Verification items for the finished model (mm, model axes). A direction names the side the tool comes from. Coordinates: 2 decimals unless noted, no trailing zeros. Order: outer loops, then holes, each group sorted by start corner. A loop starts at its lowest first (then second) coordinate and runs counter-clockwise, first axis right, second up.
Q1. Thickness scan on line 1 (X direction, y = -85, z = 5.25); line 2 (Z direction, x = -12, y = -46); line 3 (X direction, y = -49, z = 4.25). Record the ranges inside material, lowest first.
Q2. Draft check along Z on faces 1 (the flat face through (0, 48, -7.5)), 2 (the flat face through (0, -46, -0.5)), 3 (the flat face through (0, -44.031, -5)). Enter one of: pulls with the +Z half, pulls with the -Z half, needs draft (parallel to the pull), parting line crosses it, or undercut.
Q3. Depth check by flat-ended pin: P1, Ø3.5, axis at x = -7.5, y = -44, coming from the +Z side; P2, Ø2, axis at y = -70.5, z = 7, coming from the -X side; P3, Ø1, axis at x = -25.5, z = 1, coming from the -Y side. Enter the tip coordinate at first touch or a pass-through.
Q4. Cross-section at A-A, the plane y = 9.5. Record the boundary of the cut face in (x, z).
Q5. Set-up check for faces 4 (the flat face through (-17.363, 42, 0)), 5 (the cylindrical face through (-25.937, 24.446, -0.133)), 6 (the cylindrical face through (-10, 48, 0)), 7 (the flat face through (-20, -86, 0)): record each of +Z, -Z, +X, -X, +Y, -Y from which the full face is reachable in a straight line by a thin tool's end or side.
Q6. Cross-section at B-B, the plane x = 24.5. Record the boundary of the cut face in (y, z), and give its area (3 significant figures).
from build123d import *

# Parameters (mm, degrees)
BOSS_EXTRUDE1_DEPTH  = 6.9
BOSS_EXTRUDE2_START  = -6.9
BOSS_EXTRUDE2_DEPTH  = 51.9
CUT_EXTRUDE1_DEPTH   = 50.160278182
BOSS_EXTRUDE4_START  = -6.9
BOSS_EXTRUDE4_DEPTH  = 6.9
BOSS_EXTRUDE5_DEPTH  = 19
BOSS_EXTRUDE8_DEPTH  = 19
CUT_EXTRUDE2_DEPTH   = 38.1
SKETCH16_W           = 3.4
SKETCH16_H           = 19
BOSS_EXTRUDE10_DEPTH = 68.4
BOSS_EXTRUDE11_DEPTH = 68.4
SKETCH18_W           = 40
SKETCH18_H           = 19
BOSS_EXTRUDE12_DEPTH = 5
CUT_EXTRUDE3_START   = -7.338241
SKETCH20_W           = 33.2
SKETCH20_H           = 10
CUT_EXTRUDE3_DEPTH   = 7.338241
BOSS_EXTRUDE13_DEPTH = 19
FILLET1_R            = 5
SKETCH22_R           = 2
CUT_EXTRUDE4_DEPTH   = 49.030762114


with BuildPart() as part:
    # Sketch1 → Boss-Extrude1 (new body)
    with BuildSketch(Plane(origin=(0, 0, 0), x_dir=(1, 0, 0), z_dir=(0, 1, 0))):
        with BuildLine():
            ThreePointArc((7.36326441, 9.5), (12.000269064, 0), (7.36326441, -9.5))
            Line((7.36326441, -9.5), (0, -9.5))
            Line((0, -9.5), (-7.36326441, -9.5))
            ThreePointArc((-7.36326441, -9.5), (-12.000269064, 0), (-7.36326441, 9.5))
            Line((-7.36326441, 9.5), (0, 9.5))
            Line((0, 9.5), (7.36326441, 9.5))
        make_face()
        with BuildLine():
            Line((0, 7.5), (6.64, 7.5))
            ThreePointArc((6.64, 7.5), (10.000269064, 0), (6.64, -7.5))
            Line((6.64, -7.5), (0, -7.5))
            Line((0, -7.5), (-6.64, -7.5))
            ThreePointArc((-6.64, -7.5), (-10.000269064, 0), (-6.64, 7.5))
            Line((-6.64, 7.5), (0, 7.5))
        make_face(mode=Mode.SUBTRACT)
    extrude(amount=BOSS_EXTRUDE1_DEPTH)

    # Sketch2 → Boss-Extrude2 (add)
    with BuildSketch(Plane(origin=(0, 6.9, 0), x_dir=(1, 0, 0), z_dir=(0, 1, 0)).offset(BOSS_EXTRUDE2_START)):
        with BuildLine():
            Line((-7.36326441, 9.5), (-17.36326441, 9.5))
            Line((-17.36326441, 9.5), (-17.36326441, -9.5))
            Line((-17.36326441, -9.5), (-7.36326441, -9.5))
            ThreePointArc((-7.36326441, -9.5), (-12.000269064, 0), (-7.36326441, 9.5))
        make_face()
    boss_extrude2 = extrude(amount=BOSS_EXTRUDE2_DEPTH)

    # Sketch4 → Cut-Extrude1 (cut, through all)
    with BuildSketch(Plane(origin=(0, 6.9, 0), x_dir=(1, 0, 0), z_dir=(0, 1, 0))):
        with BuildLine():
            Line((-10.915369405, -4.996906494), (-8.86326441, -9.5))
            Line((-8.86326441, -9.5), (-7.36326441, -9.5))
            ThreePointArc((-7.36326441, -9.5), (-9.411139164, -7.462870557), (-10.915369405, -4.996906494))
        make_face()
        with BuildLine():
            Line((-10.915369405, 4.996906494), (-8.86326441, 9.5))
            Line((-8.86326441, 9.5), (-7.36326441, 9.5))
            ThreePointArc((-7.36326441, 9.5), (-9.411139164, 7.462870557), (-10.915369405, 4.996906494))
        make_face()
    cut_extrude1 = extrude(amount=CUT_EXTRUDE1_DEPTH, mode=Mode.SUBTRACT)

    # Mirror2: Boss-Extrude2, Cut-Extrude1 across plane
    add(boss_extrude2.mirror(Plane(origin=(0, 0, 0), x_dir=(0, 0, 1), z_dir=(1, 0, 0))))
    add(cut_extrude1.mirror(Plane(origin=(0, 0, 0), x_dir=(0, 0, 1), z_dir=(1, 0, 0))), mode=Mode.SUBTRACT)

    # Sketch6 → Boss-Extrude4 (add)
    with BuildSketch(Plane(origin=(0, 51.9, 0), x_dir=(1, 0, 0), z_dir=(0, 1, 0)).offset(BOSS_EXTRUDE4_START)):
        with BuildLine():
            Line((10.915369405, 4.996906494), (8.86326441, 9.5))
            Line((8.86326441, 9.5), (-8.86326441, 9.5))
            Line((-8.86326441, 9.5), (-10.915369405, 4.996906494))
            ThreePointArc((-10.915369405, 4.996906494), (-12.000269064, 0), (-10.915369405, -4.996906494))
            Line((-10.915369405, -4.996906494), (-8.86326441, -9.5))
            Line((-8.86326441, -9.5), (8.86326441, -9.5))
            Line((8.86326441, -9.5), (10.915369405, -4.996906494))
            ThreePointArc((10.915369405, -4.996906494), (12.000269064, 0), (10.915369405, 4.996906494))
        make_face()
        with BuildLine():
            Line((-6.64, 7.5), (6.64, 7.5))
            ThreePointArc((6.64, 7.5), (10.000269064, 0), (6.64, -7.5))
            Line((6.64, -7.5), (-6.64, -7.5))
            ThreePointArc((-6.64, -7.5), (-10.000269064, 0), (-6.64, 7.5))
        make_face(mode=Mode.SUBTRACT)
    extrude(amount=BOSS_EXTRUDE4_DEPTH)

    # Sketch7 → Boss-Extrude5 (add)
    with BuildSketch(Plane.XY.offset(9.5)):
        Polygon((-17.36326441, 31.95), (-35, 31.95), (-35, -23.05), (-27.36326441, -23.05), (-27.36326441, 25.95), (-17.36326441, 25.95), align=None)
    boss_extrude5 = extrude(amount=-BOSS_EXTRUDE5_DEPTH)

    # Mirror4: Boss-Extrude5 across plane
    add(boss_extrude5.mirror(Plane(origin=(0, 0, 0), x_dir=(0, 0, 1), z_dir=(1, 0, 0))))

    # Sketch11 → Boss-Extrude8 (add)
    with BuildSketch(Plane.XY.offset(9.5)):
        Polygon((-35, -23.05), (-20, -49.030762114), (20, -49.030762114), (35, -23.05), (27.36326441, -23.05), (15.250015756, -44.030762114), (-15.250015756, -44.030762114), (-27.36326441, -23.05), align=None)
    extrude(amount=-BOSS_EXTRUDE8_DEPTH)

    # Sketch15 → Cut-Extrude2 (cut)
    with BuildSketch(Plane(origin=(0, 6.9, 0), x_dir=(1, 0, 0), z_dir=(0, 1, 0))):
        Polygon((-12.000269064, 0), (-12.000269064, 9.5), (12.000269064, 9.5), (12.000269064, 0), (12.000269064, -9.5), (-12.000269064, -9.5), align=None)
    extrude(amount=CUT_EXTRUDE2_DEPTH, mode=Mode.SUBTRACT)

    # Sketch16 → Boss-Extrude10 (add)
    with BuildSketch(Plane.XZ.offset(49.030762114)):
        with Locations((-18.3, 0)):
            Rectangle(SKETCH16_W, SKETCH16_H)
        with Locations((18.3, 0)):
            Rectangle(SKETCH16_W, SKETCH16_H)
    extrude(amount=BOSS_EXTRUDE10_DEPTH)

    # Sketch17 → Boss-Extrude11 (add)
    with BuildSketch(Plane.XZ.offset(49.030762114)):
        with BuildLine():
            Line((-14.6, -9.5), (-16.6, -9.5))
            Line((-16.6, -9.5), (-16.6, -7.5))
            ThreePointArc((-16.6, -7.5), (-16.014213562, -8.914213562), (-14.6, -9.5))
        make_face()
        with BuildLine():
            Line((14.6, -9.5), (16.6, -9.5))
            Line((16.6, -9.5), (16.6, -7.5))
            ThreePointArc((16.6, -7.5), (16.014213562, -8.914213562), (14.6, -9.5))
        make_face()
    extrude(amount=BOSS_EXTRUDE11_DEPTH)

    # Sketch18 → Boss-Extrude12 (add)
    with BuildSketch(Plane.XZ.offset(117.430762114)):
        Rectangle(SKETCH18_W, SKETCH18_H)
    extrude(amount=BOSS_EXTRUDE12_DEPTH)

    # Sketch20 → Cut-Extrude3 (cut)
    with BuildSketch(Plane.XZ.offset(49.030762114).offset(CUT_EXTRUDE3_START)):
        with Locations((0, 4.5)):
            Rectangle(SKETCH20_W, SKETCH20_H)
    extrude(amount=CUT_EXTRUDE3_DEPTH, mode=Mode.SUBTRACT)

    # Sketch21 → Boss-Extrude13 (add)
    with BuildSketch(Plane.XY.offset(9.5)):
        Polygon((-20, -122.430762114), (0, -197.071778265), (20, -122.430762114), align=None)
    extrude(amount=-BOSS_EXTRUDE13_DEPTH)

    # Fillet1
    fillet1_edges = [part.edges().sort_by_distance(p)[0] for p in [
        (20, -122.430762114, 0),
        (20, -49.030762114, 0),
        (35, -23.05, 0),
        (35, 31.95, 0),
        (17.36326441, 31.95, 0),
        (-17.36326441, 31.95, 0),
        (-35, 31.95, 0),
        (-35, -23.05, 0),
        (-20, -49.030762114, 0),
        (-20, -122.430762114, 0),
        (-17.36326441, 0, 0),
        (17.36326441, 25.95, 0),
        (17.36326441, 0, 0),
        (17.36326441, 51.9, 0),
        (-17.36326441, 25.95, 0),
        (-17.36326441, 51.9, 0),
        (-27.36326441, -23.05, 0),
        (27.36326441, -23.05, 0),
        (27.36326441, 25.95, 0),
        (-27.36326441, 25.95, 0),
    ]]
    fillet(fillet1_edges, radius=FILLET1_R - 0.0001)  # a hair under: the kernel refuses the full size

    # Sketch22 → Cut-Extrude4 (cut)
    with BuildSketch(Plane.XZ.offset(49.030762114)):
        with Locations(Location((-12.1, -4.5, 0), (0, 0, 270))):
            Circle(SKETCH22_R)
    extrude(amount=-CUT_EXTRUDE4_DEPTH, mode=Mode.SUBTRACT)


solid = part.part
Check values:
1. line 1: x = -20 to -16.6, 16.6 to 20
1. line 2: z = -9.5 to -6.5, -2.5 to -0.5
1. line 3: x = -20.19 to -16.6, 16.6 to 20.19
2. face 1: undercut
2. face 2: pulls with the +Z half
2. face 3: needs draft
3. P1: stops at z = -0.5
3. P2: stops at x = -20
3. P3: stops at y = -40.37
4. outline: (-35, -9.5) - (-27.36, -9.5) - (-27.36, 9.5) - (-35, 9.5) - close; (-17.36, -9.5) - (-12, -9.5) - (-12, 9.5) - (-17.36, 9.5) - close; (12, -9.5) - (17.36, -9.5) - (17.36, 9.5) - (12, 9.5) - close; (27.36, -9.5) - (35, -9.5) - (35, 9.5) - (27.36, 9.5) - close
5. face 4: +Z, -Z, -X, +Y
5. face 5: +Z, -Z
5. face 6: +Y
5. face 7: +Z, -Z, -X, -Y
6. outline: (-41.24, -9.5) - (-28.01, -9.5) - (-28.01, 9.5) - (-41.24, 9.5) - close; (25.47, -9.5) - (31.95, -9.5) - (31.95, 9.5) - (25.47, 9.5) - close
6. area: 374 mm2
